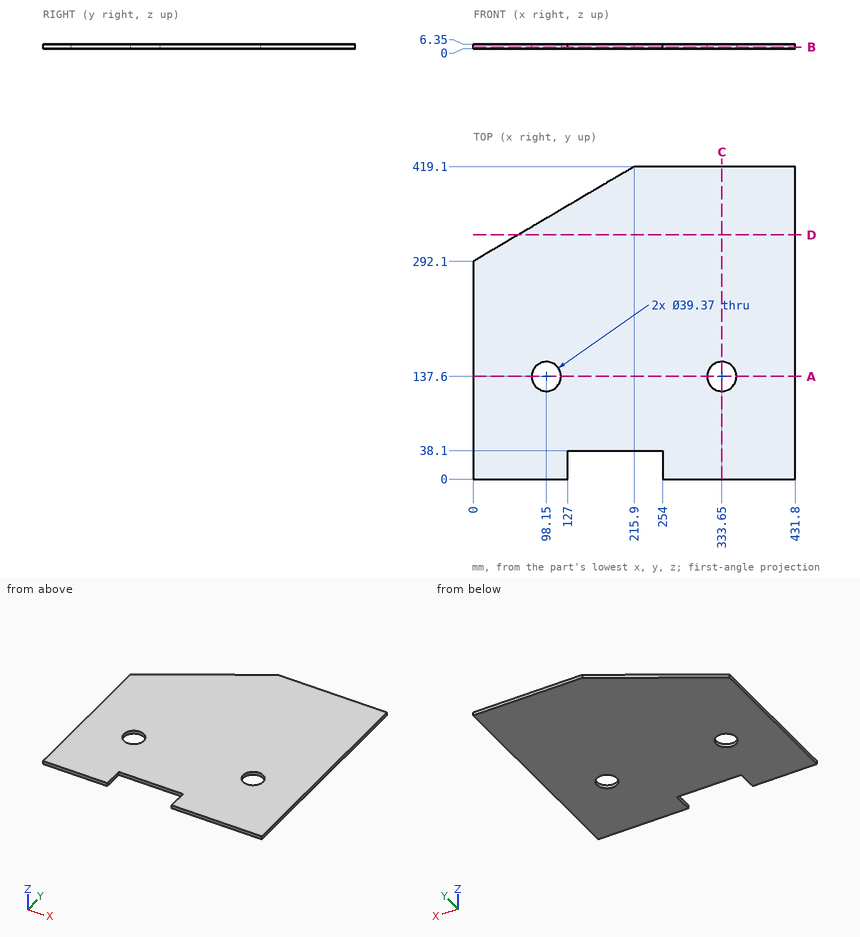
Study the drawing (mm; zero at the part's minimum x, y, z) and answer. Coordinates: 2 decimals unless noted, no trailing zeros. Write each loop counter-clockwise with the first axis right and the second up, starting at its lowest first coordinate (ties: lowest second). Pieces come first, ordered by that corner, then holes. Notation, with made-up numbers: (48, 62) - (90, 62) arc R16 cw to (90, 70) - close; hole circle Ø9 at (81.5, -33.75). An arc over 180 degrees is marked (long way). Put each result on its own line as item: value.
1. A flat-ended cylindrical pin translates along its axis: pin 1 Ø23.5 at (x, y) = (333.65, 137.6) entering from +Z. Find the tip coordinate at first contact, or state that the pin passes through.
Answer sheet:
pin 1: passes through
2. Find the intervals of material crossed by line 1 along Y through (x, z) = (333.65, 4) (3 decimals); line 2 along X through (y, z) = (27.5, 1.25); line 3 along Y through (x, z) = (253, 1), in increasing order. Write a range as from..to.
Answer sheet:
line 1: y = 0..117.915, 157.285..419.1
line 2: x = 0..127, 254..431.8
line 3: y = 38.1..419.1
3. The part is cut by section C-C on x = 333.65. Give the vertices of the cut face in (y, z) (3 decimals), plus the area to 3 significant figures.
Answer sheet:
outline: (0, 0) - (117.915, 0) - (117.915, 6.35) - (0, 6.35) - close; (157.285, 0) - (419.1, 0) - (419.1, 6.35) - (157.285, 6.35) - close
area: 2,410 mm^2
4. The part is cut by section B-B on z = 2. Give the vertices of the cut face in (x, y) (3 decimals), plus the area to 3 significant figures.
Answer sheet:
outline: (0, 0) - (127, 0) - (127, 38.1) - (254, 38.1) - (254, 0) - (431.8, 0) - (431.8, 419.1) - (215.9, 419.1) - (0, 292.1) - close; hole circle Ø39.37 at (98.15, 137.6); hole circle Ø39.37 at (333.65, 137.6)
area: 160,000 mm^2
5. The part is cut by section A-A on y = 137.6. Give the vertices of the cut face in (x, z) (3 decimals), plus the area to 3 significant figures.
Answer sheet:
outline: (0, 0) - (78.465, 0) - (78.465, 6.35) - (0, 6.35) - close; (117.835, 0) - (313.965, 0) - (313.965, 6.35) - (117.835, 6.35) - close; (353.335, 0) - (431.8, 0) - (431.8, 6.35) - (353.335, 6.35) - close
area: 2,240 mm^2
6. The part is cut by section D-D on y = 327.5. Give the vertices of the cut face in (x, z), plus the area to 3 significant figures.
Answer sheet:
outline: (60.18, 0) - (431.8, 0) - (431.8, 6.35) - (60.18, 6.35) - close
area: 2,360 mm^2
